from build123d import *

# Parameters (mm, degrees)
SKETCH_1_R          = 7.5
EXTRUDE_1_DEPTH     = 4
SKETCH_2_R          = 2.5
EXTRUDE_2_DEPTH     = 15
SKETCH_3_W          = 2
SKETCH_3_H          = 15
CUT_EXTRUDE_1_DEPTH = 2


with BuildPart() as part:
    # Эскиз1 → Бобышка-Вытянуть1 (new body)
    with BuildSketch(Plane(origin=(0, 0, 0), x_dir=(1, 0, 0), z_dir=(0, 1, 0))):
        Circle(SKETCH_1_R)
    extrude(amount=EXTRUDE_1_DEPTH)

    # Эскиз2 → Бобышка-Вытянуть2 (add)
    with BuildSketch(Plane(origin=(0, 4, 0), x_dir=(1, 0, 0), z_dir=(0, 1, 0))):
        with Locations((0, 0.136309696)):
            Circle(SKETCH_2_R)
    extrude(amount=EXTRUDE_2_DEPTH)

    # Эскиз3 → Вырез-Вытянуть1 (cut)
    with BuildSketch(Plane.XZ):
        Rectangle(SKETCH_3_W, SKETCH_3_H)
    extrude(amount=-CUT_EXTRUDE_1_DEPTH, mode=Mode.SUBTRACT)


solid = part.part
Design review of the part built by this model. Coordinates are the model's own, in mm. A direction names the side the tool comes from. Round coordinates to 2 decimals unless told otherwise and drop trailing zeros. Loops run counter-clockwise (first coordinate to the right, second up) from the corner with the lowest first, then second, coordinate; pieces in that order, holes last. Notation, with made-up numbers: (-12, -30) - (11, -30) arc R30 cw to (11, -6) - close; hole circle Ø5 at (75.5, 34). An arc over 180 degrees is marked (long way). One line per item, written item: value. Start each with the question number.
1) Consider section C-C on y = 3.75. Give the boundary of the cut face in (x, z), then the cut area to 3 significant figures.
2) To check wall thickness, follow L1, parallel to Y at x = 0.75, z = 4.75; L2, parallel to Y at x = 5, z = 1.5; L3, parallel to X at y = 1.75, z = -3. State the ranges of each line that lie inside material, in increasing order. Write a range as from..to.
3) Insertion check: pin 1 Ø1.5 at (x, y) = (4, 7.5) entering from +Z; pin 2 Ø0.6 at (x, z) = (-0.5, -3) entering from -Y; pin 3 Ø7.5 at (x, z) = (-3.5, 0) entering from +Y; pin 4 Ø1 at (x, y) = (-5, 2) entering from +Z. Each pin has a flat end and moves straight along its axis. Give the tip position at first contact, or say it passes through.
4) Consider section B-B on x = 0. Give the boundary of the cut face in (y, z).
5) Consider section A-A on z = -4.5. Give the boundary of the cut face in (x, y), then the cut area to 3 significant figures.
6) Consider section D-D on z = 1.25. Give the boundary of the cut face in (x, y), then the cut area to 3 significant figures.
7) Draft analysis for pull direction X (two halves, no side actions). For faces 4 (the cylindrical face through (2.385, 11.395, -0.887)), 5 (the flat face through (0, 2, 0)), 6 (the flat face through (3, 0, 0)), state which applies: +X half, -X half, draft (parallel to the pull), parting line (faces both ways), or undercut.
8) For faces 1 (the flat face through (1, 1, 0)), 2 (the flat face through (0, 19, 0)), 3 (the flat face through (3, 4, 0)), list the 3-axis set-ups (+Z, -Z, +X, -X, +Y, -Y) from which the entire face can be reached by the end or side of a thin tool; tool diameter is ignored.
Reported:
1. outline: circle Ø15 at (0, 0)
1. area: 177 mm^2
2. L1: y = 2..4
2. L2: y = 0..4
2. L3: x = -6.87..-1, 1..6.87
3. pin 1: passes through
3. pin 2: stops at y = 2
3. pin 3: stops at y = 19
3. pin 4: stops at z = 6
4. outline: (2, -7.5) - (4, -7.5) - (4, -2.64) - (19, -2.64) - (19, 2.36) - (4, 2.36) - (4, 7.5) - (2, 7.5) - close
5. outline: (-6, 0) - (-1, 0) - (-1, 2) - (1, 2) - (1, 0) - (6, 0) - (6, 4) - (-6, 4) - close
5. area: 44.0 mm^2
6. outline: (-7.4, 0) - (-1, 0) - (-1, 2) - (1, 2) - (1, 0) - (7.4, 0) - (7.4, 4) - (2.08, 4) - (2.08, 19) - (-2.08, 19) - (-2.08, 4) - (-7.4, 4) - close
6. area: 118 mm^2
7. face 4: parting line
7. face 5: undercut
7. face 6: draft
8. face 1: +Z, -Z, -Y
8. face 2: +Z, -Z, +X, -X, +Y
8. face 3: +Y
